Input: part model. Units: mm. Frame: model coordinates. A direction names the side the tool comes from. Coordinates: 2 decimals unless noted, no trailing zeros. Loops run counter-clockwise (first coordinate to the right, second up) from the corner with the lowest first, then second, coordinate; pieces in that order, holes last.
(1) Section D-D, the plane x = -30. Return loops of the section in (y, z).
(2) Section A-A, the plane x = -10.5. Return loops of the section in (y, z), then the cut area to 3 significant figures.
(3) Contact query for flat-ended pins moving along their axis: P1, Ø8.5, axis at x = 60, y = 52, coming from the -Z side; P2, Ø1.5, axis at y = -3.5, z = 1, coming from the +X side; P3, Ø0.9, axis at x = 54, z = 1, coming from the +Y side; P4, Ø1, axis at y = 14.5, z = 0.5, coming from the -X side. Output: stop coordinate, or through.
(4) Section C-C, the plane y = 31.5. Return loops of the section in (x, z), then the cut area to 3 significant figures.
(5) Mould query, pull axis X, two halves, no side actions, for faces 1 (the face through (-54.56, 39.23, 1.48)), 2 (the face through (-1, 60, 0)), 3 (the face through (0, 52, 2)). Classes: released by +X, released by -X, zero draft, split by the parting line, or undercut.
(6) Set-up query: faces 4 (the face through (30, -12, 1)), 5 (the face through (0, 16, 2)), 6 (the face through (25, -6, 1)). Return all of +Z, -Z, +X, -X, +Y, -Y with unobstructed straight access to the full face (end or side cutting, diameter ignored); none if empty.
(7) Line query: L1, parallel to Y at x = 5, z = 0.65; L2, parallel to Y at x = 60, z = 0.85; L3, parallel to Y at x = -30, z = 1.4. Output: solid intervals per line, ascending.
(8) Section B-B, the plane y = -7. Return loops of the section in (x, z), then the cut area to 3 significant figures.
```python
from build123d import *

# Parameters (mm, degrees)
SKETCH_1_W          = 10
SKETCH_1_H          = 20
SKETCH_1_R          = 2.6
EXTRUDE_1_DEPTH     = 3
CUT_EXTRUDE_1_DEPTH = 3
FILLET_2_R          = 3
CHAMFER_3_SIZE      = 5
CHAMFER_4_SIZE      = 5
CHAMFER_5_SIZE      = 5
SKETCH_4_R          = 2.6
CUT_EXTRUDE_2_DEPTH = 92.268833673
CHAMFER_8_SIZE      = 8
CHAMFER_9_SIZE      = 8


with BuildPart() as part:
    # 草图1 → 凸台-拉伸1 (new body)
    # profile 1 of 3: a face of its own
    with BuildSketch(Plane.XY):
        Polygon((-40, 27), (-35, 8), (-25, 8), (-25, 4), (25, 4), (25, 8), (35, 8), (40, 27), (65, 48), (65, 60), (50, 60), (24, 64), (-24, 64), (-50, 60), (-65, 60), (-65, 48), align=None)
    # profile 2 of 3: a face of its own
    with BuildSketch(Plane.XY):
        with Locations((-30, -2)):
            Rectangle(SKETCH_1_W, SKETCH_1_H)
        with Locations((-30, -7)):
            Circle(SKETCH_1_R, mode=Mode.SUBTRACT)
        with Locations((-30, 0)):
            Circle(SKETCH_1_R, mode=Mode.SUBTRACT)
    # profile 3 of 3: a face of its own
    with BuildSketch(Plane.XY):
        with Locations((30, -2)):
            Rectangle(SKETCH_1_W, SKETCH_1_H)
        with Locations((30, -7)):
            Circle(SKETCH_1_R, mode=Mode.SUBTRACT)
        with Locations((30, 0)):
            Circle(SKETCH_1_R, mode=Mode.SUBTRACT)
    extrude(amount=EXTRUDE_1_DEPTH)

    # 草图2 → 切除-拉伸1 (cut)
    with BuildSketch(Plane.XY.offset(3)):
        Polygon((-18, 52), (18, 52), (28, 42), (28, 26), (18, 16), (-18, 16), (-28, 26), (-28, 42), align=None)
    extrude(amount=-CUT_EXTRUDE_1_DEPTH, mode=Mode.SUBTRACT)

    # 圆角2
    fillet_2_edges = [part.edges().sort_by_distance(p)[0] for p in [
        (25, 4, 1.5),
        (-25, 4, 1.5),
    ]]
    fillet(fillet_2_edges, radius=FILLET_2_R)

    # 倒角3
    chamfer_3_edges = [part.edges().sort_by_distance(p)[0] for p in [
        (-40, 27, 1.5),
    ]]
    chamfer(chamfer_3_edges, length=CHAMFER_3_SIZE)

    # 倒角4
    chamfer_4_edges = [part.edges().sort_by_distance(p)[0] for p in [
        (40, 27, 1.5),
    ]]
    chamfer(chamfer_4_edges, length=CHAMFER_4_SIZE)

    # 倒角5
    chamfer_5_edges = [part.edges().sort_by_distance(p)[0] for p in [
        (-65, 60, 1.5),
        (65, 60, 1.5),
    ]]
    chamfer(chamfer_5_edges, length=CHAMFER_5_SIZE)

    # 草图4 → 切除-拉伸2 (cut, through all)
    with BuildSketch(Plane.XY.offset(3)):
        with Locations((-60, 52)):
            Circle(SKETCH_4_R)
        with Locations((-54, 46)):
            Circle(SKETCH_4_R)
        with Locations((-47, 54)):
            Circle(SKETCH_4_R)
        with Locations((-48, 40)):
            Circle(SKETCH_4_R)
        with Locations((-39, 54)):
            Circle(SKETCH_4_R)
    cut_extrude_2 = extrude(amount=-CUT_EXTRUDE_2_DEPTH, mode=Mode.SUBTRACT)

    # 镜向4: 切除-拉伸2 across plane
    add(cut_extrude_2.mirror(Plane(origin=(0, 0, 0), x_dir=(0, 0, 1), z_dir=(1, 0, 0))), mode=Mode.SUBTRACT)

    # 倒角8
    chamfer_8_edges = [part.edges().sort_by_distance(p)[0] for p in [
        (-28, 26, 1.5),
    ]]
    chamfer(chamfer_8_edges, length=CHAMFER_8_SIZE)

    # 倒角9
    chamfer_9_edges = [part.edges().sort_by_distance(p)[0] for p in [
        (28, 26, 1.5),
    ]]
    chamfer(chamfer_9_edges, length=CHAMFER_9_SIZE)


solid = part.part
```
Report:
1. outline: (-12, 0) - (-9.6, 0) - (-9.6, 3) - (-12, 3) - close; (-4.4, 0) - (-2.6, 0) - (-2.6, 3) - (-4.4, 3) - close; (2.6, 0) - (63.08, 0) - (63.08, 3) - (2.6, 3) - close
2. outline: (4, 0) - (16, 0) - (16, 3) - (4, 3) - close; (52, 0) - (64, 0) - (64, 3) - (52, 3) - close
2. area: 72.0 mm2
3. P1: stops at z = 0
3. P2: stops at x = 35
3. P3: stops at y = 60
3. P4: stops at x = -36.84
4. outline: (-45.36, 0) - (-26.96, 0) - (-26.96, 3) - (-45.36, 3) - close; (26.96, 0) - (45.36, 0) - (45.36, 3) - (26.96, 3) - close
4. area: 110 mm2
5. face 1: released by -X
5. face 2: zero draft
5. face 3: undercut
6. face 4: +Z, -Z, +X, -X, -Y
6. face 5: +Z, -Z
6. face 6: +Z, -Z, -Y
7. L1: y = 4 to 16, 52 to 64
7. L2: y = 43.8 to 49.4, 54.6 to 60
7. L3: y = -12 to -9.6, -4.4 to -2.6, 2.6 to 63.08
8. outline: (-35, 0) - (-32.6, 0) - (-32.6, 3) - (-35, 3) - close; (-27.4, 0) - (-25, 0) - (-25, 3) - (-27.4, 3) - close; (25, 0) - (27.4, 0) - (27.4, 3) - (25, 3) - close; (32.6, 0) - (35, 0) - (35, 3) - (32.6, 3) - close
8. area: 28.8 mm2
